For this review, take the finished solid that the model builds, in its own axes (mm). Coordinates: 2 decimals unless noted, no trailing zeros. Write each loop counter-clockwise with the first axis right and the second up, starting at its lowest first coordinate (ties: lowest second). Pieces come first, ordered by that corner, then holes. Notation, with made-up numbers: (5.25, 14.25) - (59.25, 14.25) arc R12 ccw to (59.25, 31.25) - close; hole circle Ø4 at (24, 48.25). An arc over 180 degrees is marked (long way). Use one line per item in the form item = value. Start each with the question number.
1) We need section A-A (y = 300). Give the boundary of the cut face in (x, z).
2) We need section C-C (y = 265.5). Give the boundary of the cut face in (x, z), plus the area to 3 significant figures.
3) We need section D-D (x = 4.5). Give the boundary of the cut face in (y, z).
4) We need section B-B (z = 286.5). Give the boundary of the cut face in (x, y).
5) Insertion check: P1, Ø10.5, axis at y = 267.33, z = 321.08, coming from the -X side; P2, Ø3, axis at x = 1, z = 263.5, coming from the +Y side; P3, Ø1.5, axis at x = 3.5, y = 315, coming from the -Z side; P4, Ø4, axis at y = 253.43, z = 241.1, coming from the -X side (1 decimal). Each pin has a flat end and moves straight along its axis. Give the tip position at first contact, or say it passes through.
6) For L1, parallel to Z at x = 5, y = 291.5; L2, parallel to Z at x = 5.5, y = 286; L3, parallel to Y at x = 5, z = 240.5, list the stretches that pass through material, from the lowest coordinate up. Write a range as from..to.
Autodesk Inventor part; units mm, degrees
ref_plane "YZ Plane" through (0, 0, 0) normal (1, 0, 0) x (0, 1, 0)
ref_plane "XZ Plane" through (0, 0, 0) normal (0, 1, 0) x (-1, 0, 0)
ref_plane "XY Plane" through (0, 0, 0) normal (0, 0, 1) x (1, 0, 0)
sketch "Sketch1" plane through (0, 0, 0) normal (1, 0, 0) x (0, 1, 0)
  line L0 (95.25, 812.8) -> (44.45, 812.8) construction
  line L1 (44.45, 812.8) -> (44.45, 0) construction
  line L2 (44.45, 0) -> (95.25, 0) construction
  line L3 (95.25, 0) -> (95.25, 812.8) construction
  line L4 (95.25, 0) -> (44.45, 0) construction
  line L5 (44.45, 25.4) -> (95.25, 25.4) construction
  circle A0 centre (190.5, 0) radius 50.8 construction
  circle A1 centre (95.25, 279.4) radius 25.4 construction
  circle A2 centre (274.9493, 279.9916) radius 9.525 construction
  circle A3 centre (274.9493, 279.9916) radius 25.4 construction
  circle A4 centre (274.9493, 279.9916) radius 31.75 construction
  circle A5 centre (609.6, 438.15) radius 50.8 construction
  circle A6 centre (274.9493, 279.9916) radius 30.48 construction
  circle A7 centre (587.8333, 365.125) radius 25.4 construction
  circle A8 centre (587.8333, 511.175) radius 25.4 construction
  line L6 (587.8333, 485.775) -> (587.8333, 390.525) construction
  circle A9 centre (490.3356, 512.7625) radius 14.351 construction
  circle A10 centre (392.825, 512.7625) radius 14.351 construction
  circle A11 centre (490.3356, 363.5375) radius 14.351 construction
  line L7 (587.8333, 511.175) -> (490.3356, 512.7625) construction
  line L8 (587.8333, 365.125) -> (490.3356, 363.5375) construction
  circle A12 centre (490.3356, 512.7625) radius 25.4 construction
  circle A13 centre (490.3356, 363.5375) radius 25.4 construction
  line L9 (490.3356, 487.3625) -> (490.3356, 388.9375) construction
  circle A14 centre (392.825, 512.7625) radius 25.4 construction
  circle A15 centre (392.825, 363.5375) radius 25.4 construction
  circle A16 centre (392.825, 363.5375) radius 14.351 construction
  line L10 (490.3356, 512.7625) -> (392.825, 512.7625) construction
  line L11 (490.3356, 363.5375) -> (392.825, 363.5375) construction
  line L12 (392.825, 487.3625) -> (392.825, 388.9375) construction
  circle A17 centre (295.3189, 511.8309) radius 25.4 construction
  circle A18 centre (295.3189, 362.6059) radius 25.4 construction
  circle A19 centre (203.1597, 479.9719) radius 25.4 construction
  circle A20 centre (295.3189, 511.8309) radius 14.351 construction
  circle A21 centre (295.3189, 362.6059) radius 14.351 construction
  circle A22 centre (203.1597, 479.9719) radius 14.351 construction
  line L13 (392.825, 512.7625) -> (295.3189, 511.8309) construction
  line L14 (392.825, 363.5375) -> (295.3189, 362.6059) construction
  line L15 (295.3189, 486.4309) -> (295.3189, 388.0059) construction
  line L16 (295.3189, 511.8309) -> (203.1597, 479.9719) construction
  circle A23 centre (123.1487, 424.2353) radius 25.4 construction
  circle A24 centre (123.1487, 424.2353) radius 14.351 construction
  line L17 (203.1597, 479.9719) -> (123.1487, 424.2353) construction
  circle A25 centre (95.25, 279.4) radius 14.351 construction
  line L18 (609.6, 355.6) -> (44.45, 355.6) construction
  line L19 (44.45, 355.6) -> (44.45, 330.2) construction
  line L20 (44.45, 330.2) -> (609.6, 330.2) construction
  line L21 (609.6, 330.2) -> (609.6, 355.6) construction
  line L22 (95.25, 241.3) -> (44.45, 241.3) construction
  line L23 (44.45, 241.3) -> (44.45, 215.9) construction
  line L24 (44.45, 215.9) -> (95.25, 215.9) construction
  line L25 (95.25, 215.9) -> (95.25, 241.3) construction
  circle A26 centre (244.475, 279.4) radius 25.4 construction
  circle A27 centre (244.475, 279.4) radius 14.351 construction
  line L26 (218.8463, 459.9947) -> (279.6322, 382.5831) construction
  circle A28 centre (274.9493, 279.9916) radius 8.89 construction
  circle A29 centre (288.401, 252.6405) radius 21.59 construction
  circle A30 centre (244.475, 279.4) radius 21.59 construction
  circle A31 centre (288.401, 252.6405) radius 14.351
  circle A32 centre (587.8333, 511.175) radius 14.351 construction
  circle A33 centre (587.8333, 365.125) radius 14.351 construction
  line L27 (95.25, 647.7) -> (609.6, 647.7) construction
  line L28 (609.6, 647.7) -> (609.6, 622.3) construction
  line L29 (609.6, 622.3) -> (95.25, 622.3) construction
  line L30 (95.25, 622.3) -> (95.25, 647.7) construction
  circle A34 centre (600.5333, 552.45) radius 3.2639 construction
  circle A35 centre (600.5333, 552.45) radius 6.35 construction
  circle A36 centre (600.5333, 336.55) radius 3.2639 construction
  circle A37 centre (600.5333, 336.55) radius 6.35 construction
  circle A38 centre (114.3, 552.45) radius 3.2639 construction
  circle A39 centre (114.3, 552.45) radius 6.35 construction
  line L31 (595.3031, 535.4518) -> (598.6659, 546.3808) construction
  circle A40 centre (63.5, 264.8503) radius 3.2639 construction
  circle A41 centre (63.5, 264.8503) radius 6.35 construction
  line L32 (337.9424, 330.2) -> (600.5333, 330.2) construction
  circle A42 centre (288.401, 252.6405) radius 24.13 construction
  circle A43 centre (244.475, 279.4) radius 24.13 construction
  line L33 (72.1591, 268.8184) -> (69.2727, 267.4957) construction
  line L34 (609.6, 342.9) -> (44.45, 342.9) construction
  line L35 (265.0822, 266.8462) -> (267.7937, 265.1944) construction
  circle A44 centre (318.8924, 273.2978) radius 3.2639
  circle A45 centre (253.4257, 241.1003) radius 3.2639
  line L36 (95.25, 558.8) -> (44.45, 558.8) construction
  line L37 (44.45, 558.8) -> (44.45, 533.4) construction
  line L38 (44.45, 533.4) -> (95.25, 533.4) construction
  line L39 (95.25, 533.4) -> (95.25, 558.8) construction
  line L40 (114.3, 558.8) -> (600.5333, 558.8) construction
  line L41 (108.0468, 553.5545) -> (57.2468, 265.9549) construction
  line L42 (285.1949, 228.7245) -> (62.6563, 258.5566) construction
  circle A46 centre (318.8924, 273.2978) radius 6.35 construction
  circle A47 centre (253.4257, 241.1003) radius 6.35 construction
  arc A48 (114.3, 558.8) -> (108.0468, 553.5545) centre (114.3, 552.45) ccw construction
  arc A49 (57.2468, 265.9549) -> (62.6563, 258.5566) centre (63.5, 264.8503) ccw construction
  line L43 (312.6148, 274.2541) -> (306.3372, 275.2103) construction
  line L44 (313.6352, 269.7362) -> (308.3781, 266.1746) construction
  line L45 (259.4559, 243.09) -> (265.4861, 245.0797) construction
  line L46 (256.5005, 246.6562) -> (259.5753, 252.2121) construction
  line L47 (325.2424, 317.5) -> (325.2424, 273.2978) construction
  arc A50 (337.9424, 330.2) -> (325.2424, 317.5) centre (337.9424, 317.5) ccw construction
  line L48 (324.5494, 270.4133) -> (309.8976, 241.6792) construction
  arc A51 (324.5494, 270.4133) -> (325.2424, 273.2978) centre (318.8924, 273.2978) ccw construction
  arc A52 (285.1949, 228.7245) -> (309.8976, 241.6792) centre (288.401, 252.6405) ccw construction
  circle A53 centre (431.8, 342.9) radius 3.2639 construction
  circle A54 centre (457.2, 342.9) radius 3.2639 construction
  circle A55 centre (520.7, 342.9) radius 3.2639 construction
  circle A56 centre (546.1, 342.9) radius 3.2639 construction
  line L49 (606.8833, 552.45) -> (606.8833, 336.55) construction
  arc A57 (606.8833, 552.45) -> (600.5333, 558.8) centre (600.5333, 552.45) ccw construction
  arc A58 (600.5333, 330.2) -> (606.8833, 336.55) centre (600.5333, 336.55) ccw construction
  circle A59 centre (184.15, 304.8) radius 3.2639 construction
  circle A60 centre (158.75, 304.8) radius 3.2639 construction
  circle A61 centre (133.35, 304.8) radius 3.2639 construction
  circle A62 centre (133.35, 279.4) radius 3.2639 construction
  circle A63 centre (158.75, 279.4) radius 3.2639 construction
  circle A64 centre (184.15, 279.4) radius 3.2639 construction
  circle A65 centre (289.5545, 295.8051) radius 21.59 construction
  line L50 (313.8542, 277.163) -> (306.6842, 282.6636) construction
  circle A66 centre (289.5545, 295.8051) radius 14.351
  circle A67 centre (267.3295, 321.0778) radius 3.2639
  circle A68 centre (267.3295, 321.0778) radius 6.35 construction
  circle A69 centre (289.5545, 295.8051) radius 24.13 construction
  line L51 (271.5229, 316.3094) -> (273.6196, 313.9252) construction
  line L52 (252.257, 234.8587) -> (283.9601, 228.9227)
  line L53 (324.5494, 270.4133) -> (309.8976, 241.6792)
  arc A70 (283.9601, 228.9227) -> (309.8976, 241.6792) centre (288.401, 252.6405) ccw
  line L54 (247.1695, 242.1879) -> (261.0733, 322.1654)
  line L55 (269.1628, 327.1574) -> (296.521, 318.9076)
  line L56 (324.7039, 275.8568) -> (311.6384, 305.5292)
  arc A71 (311.6384, 305.5292) -> (296.521, 318.9076) centre (289.5545, 295.8051) ccw
  arc A72 (324.5494, 270.4133) -> (324.7039, 275.8568) centre (318.8924, 273.2978) ccw
  arc A73 (269.1628, 327.1574) -> (261.0733, 322.1654) centre (267.3295, 321.0778) ccw
  arc A74 (247.1695, 242.1879) -> (252.257, 234.8587) centre (253.4257, 241.1003) ccw
  point P0 (0, 0)
  point P1 (241.139, 234.6303)
  point P2 (100.4185, 253.4945)
  dimension "d9" = 50.8
  dimension "d38" = 50.8
  dimension "d53" = 50.8
  dimension "d178" = 43.18
  dimension "d1" = 812.8
  dimension "d2" = 44.45
  dimension "d4" = 25.4
  dimension "d5" = 101.6
  dimension "d6" = 95.25
  dimension "d8" = 50.8
  dimension "d14" = 50.8
  dimension "d15" = 63.5
  dimension "d21" = 19.05
  dimension "d29" = 438.15
  dimension "d30" = 514.35
  dimension "d36" = 60.96
  dimension "d39" = 50.8
  dimension "d41" = 95.25
  dimension "d45" = 28.702
  dimension "d47" = 97.5106
  dimension "d48" = 98.425
  dimension "d56" = 25.4
  dimension "d73" = 50.8
  dimension "d74" = 25.4
  dimension "d75" = 215.9
  dimension "d78" = 279.4
  dimension "d80" = 149.225
  dimension "d81" = 97.5106
  dimension "d82" = 147.4978
  dimension "d83" = 17.78
  dimension "d85" = 43.18
  dimension "d92" = 330.2
  dimension "d100" = 514.35
  dimension "d107" = 25.4
  dimension "d108" = 514.35
  dimension "d109" = 266.7
  dimension "d115" = 6.5278
  dimension "d116" = 12.7
  dimension "d122" = 2.54
  dimension "d123" = 2.54
  dimension "d128" = 3.175
  dimension "d134" = 3.175
  dimension "d135" = 194.9958
  dimension "d136" = 6.5278
  dimension "d137" = 25.4
  dimension "d138" = 533.4
  dimension "d139" = 19.05
  dimension "d140" = 19.05
  dimension "d141" = 12.7
  dimension "d142" = 6.35
  dimension "d143" = 12.7
  dimension "d144" = 43.18
  dimension "d149" = 25.4
  dimension "d151" = 6.5278
  dimension "d157" = 25.4
  dimension "d158" = 63.5
  dimension "d159" = 12.7
  dimension "d161" = 11.4347
  dimension "d163" = 44.45
  dimension "d164" = 38.1
  dimension "d166" = 336.55
  dimension "d167" = 25.4
  dimension "d168" = 6.5278
  dimension "d169" = 25.4
  dimension "d170" = 25.4
  dimension "d173" = 25.4
  dimension "d174" = 38.1
  dimension "d175" = 25.4
extrude "Extrusion2" add sketch "Sketch1" along normal blind 6.35
properties part number "INDX_012_OuterPlate" material "Polycarbonate, Clear"
Determined:
q1.outline = (0, 231.48) - (6.35, 231.48) - (6.35, 244.19) - (0, 244.19) - close; (0, 261.09) - (6.35, 261.09) - (6.35, 285.96) - (0, 285.96) - close; (0, 305.65) - (6.35, 305.65) - (6.35, 317.56) - (0, 317.56) - close
q2.outline = (0, 232.38) - (6.35, 232.38) - (6.35, 318.37) - (0, 318.37) - close; (0, 323.78) - (6.35, 323.78) - (6.35, 327.16) - (0, 327.16) - close
q2.area = 568 mm²
q3.outline = (247.17, 242.19) arc R6.35 ccw to (252.26, 234.86) - (283.96, 228.92) arc R24.13 ccw to (309.9, 241.68) - (324.55, 270.41) arc R6.35 ccw to (324.7, 275.86) - (311.64, 305.53) arc R24.13 ccw to (296.52, 318.91) - (269.16, 327.16) arc R6.35 ccw to (261.07, 322.17) - close; hole circle Ø6.53 at (253.43, 241.1); hole circle Ø6.53 at (267.33, 321.08); hole circle Ø28.7 at (288.4, 252.64); hole circle Ø28.7 at (289.55, 295.81); hole circle Ø6.53 at (318.89, 273.3)
q4.outline = (0, 254.87) - (6.35, 254.87) - (6.35, 278.63) - (0, 278.63) - close; (0, 300.48) - (6.35, 300.48) - (6.35, 320.02) - (0, 320.02) - close
q5.P1 = 0
q5.P2 = 321.79
q5.P3 = 250.21
q5.P4 = through
q6.L1 = 228.71..238.63, 266.65..281.59, 310.02..320.42
q6.L2 = 228.63..238.49, 266.79..281.9, 309.71..322.08
q6.L3 = 247.1..250.22, 256.63..280.75, 296.05..309.25
